Build history of the part. All positions in model axes, mm. Face numbers are marked on the shaded views. A direction names the side the tool comes from. Coordinates: 2 decimals unless noted, no trailing zeros. Order: outer loops, then holes, each group sorted by start corner. A loop starts at its lowest first (then second) coordinate and runs counter-clockwise, first axis right, second up. Notation, with made-up numbers: M 49.25,61 L 101.25,61 A27 cw 101.25,87 Z; hole C -17.5,-13 d3. An arc over 180 degrees is marked long. Write item = value, one per line. Start each with the question number.
Q1. Band-saw the part on B-B on z = 0. Write the cut outline in (x, y).
Q2. Band-saw the part on D-D on x = 6. Write the cut outline in (y, z), plus the area to 3 significant figures.
Q3. Pin check, flat tips, straight feed: P1, Ø4, axis at x = -3.5, y = -3, coming from the -Z side (3 decimals); P2, Ø3, axis at x = 1, y = -3.5, coming from the +Z side; P3, Ø1, axis at y = 0.5, z = -1.5, coming from the -X side. Stop position of each tip, or through.
Q4. 3-axis set-ups, long thin cutter, end or side, ignore diameter. For the marked faces 1 and 2: which of +Z, -Z, +X, -X, +Y, -Y reach the whole face in a straight line?
Q5. Pull direction Y, two halves, no side cores. Call the marked faces 3, 4 and 5: released by +Y, released by -Y, zero draft, split by the parting line, or undercut.
Q6. Drill centre lines: probe 1 along X at (y, z) = (1, 0); probe 2 along X at (y, z) = (-4.75, 2.5); probe 3 along Z at (x, y) = (-2.75, -2.25). Where is each one in solid material? Low to high.
Q7. Band-saw the part on C-C on x = -0.25. Write the cut outline in (y, z).
Q8. Band-saw the part on A-A on x = -2.75. Write the cut outline in (y, z).
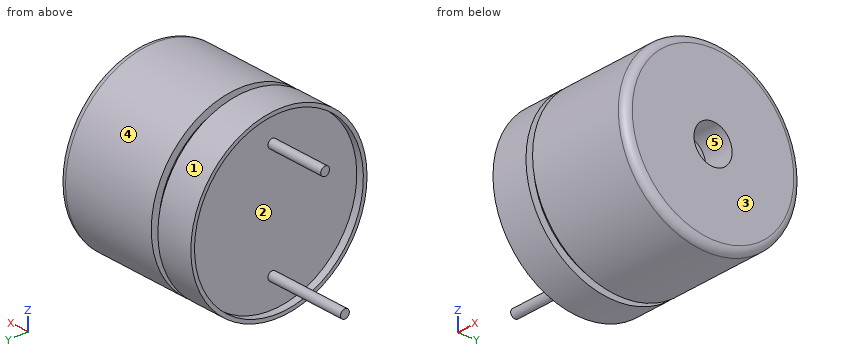
Autodesk Inventor part; units mm, degrees
ref_plane "YZ Plane" through (0, 0, 0) normal (1, 0, 0) x (0, 1, 0)
ref_plane "XZ Plane" through (0, 0, 0) normal (0, 1, 0) x (-1, 0, 0)
ref_plane "XY Plane" through (0, 0, 0) normal (0, 0, 1) x (1, 0, 0)
sketch "Sketch1" plane through (0, 0, 0) normal (0, 0, 1) x (1, 0, 0)
  point P0 (0, 0)
sketch "Sketch2" plane through (0, 0, 0) normal (0, 0, 1) x (1, 0, 0)
  line L0 (0, 0) -> (7, 0)
  line L1 (7, 0) -> (7, 6)
  line L2 (7, 6) -> (0, 6)
  line L3 (0, 6) -> (0, 0)
  line L4 (0, 0) -> (-0.5, 0)
  line L5 (-0.5, 0) -> (-0.5, 5.5)
  line L6 (-0.5, 5.5) -> (0, 5.5)
  line L7 (0, 5.5) -> (0, 0)
  line L8 (-0.5, 0) -> (-3, 0)
  line L9 (-3, 0) -> (-3, 6)
  line L10 (-3, 6) -> (-0.5, 6)
  line L11 (-0.5, 6) -> (-0.5, 0)
revolve "Revolution1" add sketch "Sketch2" angle 360 about axis through (0, 0, 0) along (1, 0, 0)
sketch "Sketch3" plane through (-3, 0, 0) normal (-1, 0, 0) x (0, 0, 1)
  circle A0 centre (0, 0) radius 5.75
  dimension "d6" = 11.5
extrude "Extrusion1" cut sketch "Sketch3" against normal blind 0.5
sketch "Sketch4" plane through (-2.5, 0, 0) normal (-1, 0, 0) x (0, 0, 1)
  line L0 (0, 0) -> (3.8, 0)
  circle A0 centre (3.8, 0) radius 0.3
  dimension "d9" = 3.8
  dimension "d10" = 0.6
extrude "Extrusion2" add sketch "Sketch4" along normal blind 4
sketch "Sketch5" plane through (-2.5, 0, 0) normal (-1, 0, 0) x (0, 0, 1)
  line L0 (0, 0) -> (-3.8, 0)
  circle A0 centre (-3.8, 0) radius 0.3
  dimension "d13" = 3.8
  dimension "d14" = 0.6
extrude "Extrusion3" add sketch "Sketch5" along normal blind 5.5
sketch "Sketch6" plane through (7, 0, 0) normal (1, 0, 0) x (0, 0, -1)
  circle A0 centre (0, 0) radius 1.3
  dimension "d17" = 2.6
extrude "Extrusion4" cut sketch "Sketch6" against normal blind 2
fillet "Fillet1" radius 0.5 1 edges at (7, -6, 0)
properties part number "buzzer"
Recorded:
q1.outline = M -3,-6 L -0.5,-6 L -0.5,-5.5 L 0,-5.5 L 0,-6 L 6.5,-6 A0.5 ccw 7,-5.5 L 7,-1.3 L 5,-1.3 L 5,1.3 L 7,1.3 L 7,5.5 A0.5 ccw 6.5,6 L 0,6 L 0,5.5 L -0.5,5.5 L -0.5,6 L -3,6 L -3,5.75 L -2.5,5.75 L -2.5,-5.75 L -3,-5.75 Z
q2.outline = C 0,0 d12; hole C 0,0 d2.6
q2.area = 108 mm2
q3.P1 = -5.905
q3.P2 = 5.66
q3.P3 = -2.5
q4.face_1 = +X, -X
q4.face_2 = -X
q5.face_3 = zero draft
q5.face_4 = split by the parting line
q5.face_5 = undercut
q6.probe_1 = -2.5 to 5
q6.probe_2 = -2.5 to 7
q6.probe_3 = -5.56 to -5.29, 5.29 to 5.56
q7.outline = C 0,0 d11
q8.outline = C 0,0 d12; C 0,-3.8 d0.6; C 0,3.8 d0.6; hole C 0,0 d11.5
